Autodesk Inventor part; units mm, degrees
ref_plane "YZ Plane" through (0, 0, 0) normal (1, 0, 0) x (0, 1, 0)
ref_plane "XZ Plane" through (0, 0, 0) normal (0, 1, 0) x (-1, 0, 0)
ref_plane "XY Plane" through (0, 0, 0) normal (0, 0, 1) x (1, 0, 0)
ref_plane "Work Plane1" through (0, 0, 0) normal (0, 0, 1) x (1, 0, 0)
sketch "Sketch1" plane through (0, 0, 0) normal (0, 0, 1) x (1, 0, 0)
  line L0 (93, -160) -> (85, -152)
  line L1 (150, -160) -> (93, -160)
  line L2 (150, -27.5) -> (150, -160)
  line L3 (110, -27.5) -> (150, -27.5)
  line L4 (110, 47.5) -> (110, -27.5)
  line L5 (150, 47.5) -> (110, 47.5)
  line L6 (150, 160) -> (150, 47.5)
  line L7 (-150, 160) -> (150, 160)
  line L8 (-150, 47.5) -> (-150, 160)
  line L9 (-110, 47.5) -> (-150, 47.5)
  line L10 (-110, -27.5) -> (-110, 47.5)
  line L11 (-150, -27.5) -> (-110, -27.5)
  line L12 (-150, -160) -> (-150, -27.5)
  line L13 (-93, -160) -> (-150, -160)
  line L14 (-85, -152) -> (-93, -160)
  line L15 (-85, -140) -> (-85, -152)
  line L16 (85, -140) -> (-85, -140)
  line L17 (85, -152) -> (85, -140)
  line L18 (-150, -280.0045) -> (150, -280.0045)
  line L19 (150, -280.0045) -> (150, -118.8161)
  line L20 (150, -118.8161) -> (-150, -118.8161)
  line L21 (-150, -118.8161) -> (-150, -280.0045)
  point P0 (0, 0)
extrude "Extrusion1" add sketch "Sketch1" against normal blind 3 contours L1 L19 L18 L21 L13 L14 L15 L16 L17 L0
sketch "Sketch2" plane through (0, 0, -3) normal (0, 0, -1) x (-1, 0, 0)
  line L0 (-149, -279.3573) -> (-149, -162.5589)
  line L1 (-79, -279.1787) -> (-149, -279.1787)
  line L2 (-149, -279.1787) -> (147.9655, -279.1787)
  line L3 (147.9655, -279.1787) -> (147.9655, -183.5488)
  line L4 (147.9655, -183.5488) -> (-149, -183.5488)
  line L5 (-149, -183.5488) -> (-149, -279.1787)
  point P0 (0, 0)
  point P1 (-149, -183.5488)
extrude "Extrusion2" add sketch "Sketch2" along normal blind 25.4
sketch "Sketch3" plane through (0, 0, -28.4) normal (0, 0, -1) x (-1, 0, 0)
  line L0 (75.5, -193.4434) -> (-74.5, -193.4434)
  line L1 (-74.5, -193.4434) -> (-74.5, -316.9258)
  line L2 (-74.5, -316.9258) -> (75.5, -316.9258)
  line L3 (75.5, -316.9258) -> (75.5, -193.4434)
  line L4 (63.5, -304.9759) -> (-62.5, -304.9759)
  line L5 (-62.5, -304.9759) -> (-62.5, -205.3933)
  line L6 (-62.5, -205.3933) -> (63.5, -205.3933)
  line L7 (63.5, -205.3933) -> (63.5, -304.9759)
  line L8 (-78.5724, -320.9982) -> (-78.5724, -189.371)
  line L9 (-78.5724, -189.371) -> (79.5724, -189.371)
  line L10 (79.5724, -189.371) -> (79.5724, -320.9982)
  line L11 (79.5724, -320.9982) -> (-78.5724, -320.9982)
  point P0 (0, 0)
extrude "Extrusion3" cut sketch "Sketch3" against normal blind 50.8 contours L3 L2 L1 L0 | L4 L5 L6 L7 | L8 L9 L10 L11
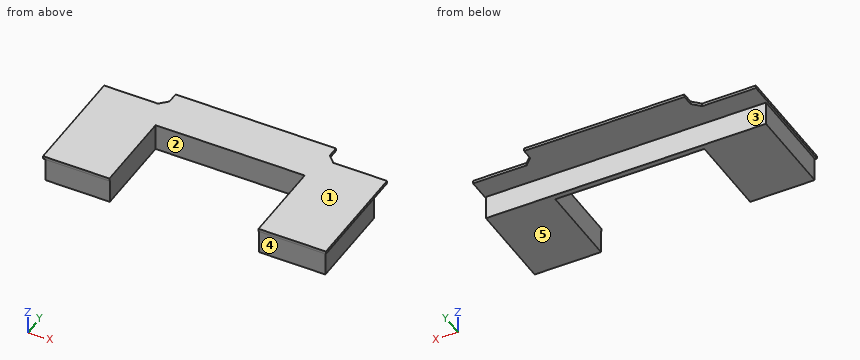
Geometry check sheet. Reference: the model listing, model coordinates, mm. Face numbers are marked on the shaded views. A direction names the side the tool comes from. Give positions to 0.01 mm unless a question says otherwise; leave off trailing zeros. Order: outer loops, then holes, each group sorted by start corner. A loop starts at its lowest first (then second) coordinate and runs counter-clockwise, first axis right, second up.
1) Gauge pin test, flat ends, axial feed: pin 1 (14 mm diameter, centred on x = -30.5, z = -18.5, fed in from -Y); pin 2 (2 mm diameter, centred on y = -221, z = -9, fed in from +X); pin 3 (8 mm diameter, centred on x = -74.5, z = -21, fed in from +Y). Record the tip position at first contact, or that the pin passes through.
Results are:
pin 1: stops at y = -189.37
pin 2: stops at x = 149
pin 3: stops at y = -183.55
2) Cross-section at A-A (y = -240). Record the boundary of the cut face in (x, z), then the cut area to 3 significant figures.
Results are:
outline: (-150, -3) - (-147.97, -3) - (-147.97, -28.4) - (-79.57, -28.4) - (-79.57, 0) - (-150, 0) - close; (78.57, -28.4) - (149, -28.4) - (149, -3) - (150, -3) - (150, 0) - (78.57, 0) - close
area: 3,950 mm2
3) Cross-section at B-B (z = -16.25). Record the boundary of the cut face in (x, y).
Results are:
outline: (-147.97, -279.18) - (-79.57, -279.18) - (-79.57, -189.37) - (78.57, -189.37) - (78.57, -279.18) - (149, -279.18) - (149, -183.55) - (-147.97, -183.55) - close
4) Cross-section at D-D (y = -171.5). Record the boundary of the cut face in (x, z).
Results are:
outline: (-150, -3) - (150, -3) - (150, 0) - (-150, 0) - close
5) Material ranges on probe 1 along X at (y, z) = (-232, -21.75); probe 2 along X at (y, z) = (-203.5, -2.25); probe 3 along Y at (x, z) = (-107, -25.75), recorded low to high.
Results are:
probe 1: x = -147.97 to -79.57, 78.57 to 149
probe 2: x = -150 to -79.57, 78.57 to 150
probe 3: y = -279.18 to -183.55
6) Tool access check on the marked faces 1, 2, 3, 4 and 5. Record the directions out of +Z, -Z, +X, -X, +Y, -Y that give a thin tool (end or side, any length) a straight path to the whole face; none if there is none.
Results are:
face 1: +Z, +X, -X, +Y, -Y
face 2: +Z, -Z, -Y
face 3: -Z, +X, -X, +Y
face 4: -Z, +X, -X, -Y
face 5: -Z, +X, -X, +Y, -Y
7) Cross-section at C-C (x = 47). Record the boundary of the cut face in (y, z).
Results are:
outline: (-189.37, -28.4) - (-183.55, -28.4) - (-183.55, -3) - (-140, -3) - (-140, 0) - (-189.37, 0) - close
